Work out the finished part from the listing and answer in its coordinate system (mm). Face numbers are marked on the shaded views. A direction names the side the tool comes from. Coordinates: 2 decimals unless noted, no trailing zeros. Use a Markdown table: item, result.
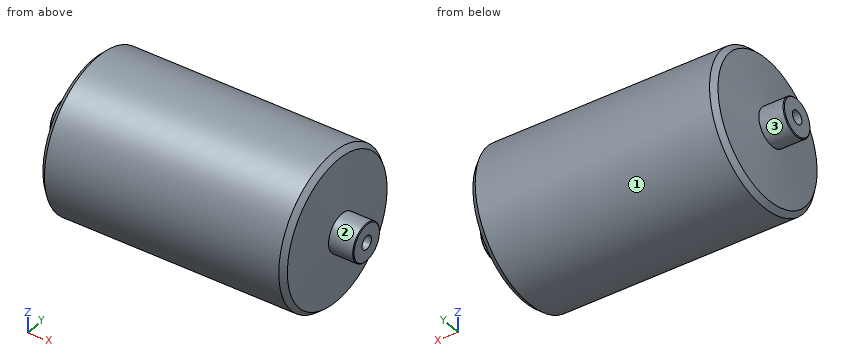
from build123d import *
from OCP.BRepFilletAPI import BRepFilletAPI_MakeChamfer

# Parameters (mm, degrees)
SKETCH_1_W       = 16.4
SKETCH_1_H       = 12.5
SKETCH_1_W_2     = 16.5
CHAMFER_1_SIZE   = 0.5
CHAMFER_2_SIZE   = 3
CHAMFER_2_SIZE2  = 3.300188603
M10X1_25_1_D     = 8.8
M10X1_25_1_DEPTH = 59
M10X1_25_1_TIP   = 2.643786724
M10X1_25_2_D     = 8.8
M10X1_25_2_DEPTH = 59
M10X1_25_2_TIP   = 2.643786724


with BuildPart() as part:
    # 草圖1 → 旋轉1 (revolve)
    with BuildSketch(Plane.XY, mode=Mode.PRIVATE) as revolve_1_sk:
        Polygon((16.5, 12.5), (16.5, 0), (183.6, 0), (183.6, 12.5), (183.6, 50), (16.5, 50), align=None)
        with Locations((191.8, 6.25)):
            Rectangle(SKETCH_1_W, SKETCH_1_H)
        with Locations((8.25, 6.25)):
            Rectangle(SKETCH_1_W_2, SKETCH_1_H)
    revolve(revolve_1_sk.sketch.rotate(Axis((16.5, 0, 0), (1, 0, 0)), 90), axis=Axis((16.5, 0, 0), (1, 0, 0)))

    # 草圖2 → 除料-旋轉1 (revolve, cut)
    with BuildSketch(Plane.XY, mode=Mode.PRIVATE) as cut_revolve_1_sk:
        Polygon((186.873055919, 74.843370729), (1.025224849, 63.173855755), (0, 12.5), (16.5, 12.5), (20.558049953, 58.883723216), (178.981866404, 65.285508546), (183.6, 12.5), (200, 12.5), align=None)
    revolve(cut_revolve_1_sk.sketch.rotate(Axis((0, 0, 0), (-1, 0, 0)), 270), axis=Axis((0, 0, 0), (-1, 0, 0)), mode=Mode.SUBTRACT)

    # 導角1
    chamfer_1_edges = [part.edges().sort_by_distance(p)[0] for p in [
        (200, 0, -12.5),
        (0, 0, -12.5),
    ]]
    chamfer(chamfer_1_edges, length=CHAMFER_1_SIZE)

    # 導角2: one chamfer whose edges measure the first distance from different faces: ONE call of the kernel's chamfer builder (chamfer() names one face for all edges)
    chamfer_2_edges_1 = [part.edges().sort_by_distance(p)[0] for p in [
        (19.780824882, 0, -50),
    ]]
    chamfer_2_side_1 = [part.faces().sort_by_distance(p)[0] for p in [
        (100.05, 0, -50),
    ]]
    chamfer_2_edges_2 = [part.edges().sort_by_distance(p)[0] for p in [
        (180.319175118, 0, -50),
    ]]
    chamfer_2_side_2 = [part.faces().sort_by_distance(p)[0] for p in [
        (181.959587559, 0, -31.25),
    ]]
    chamfer_2 = BRepFilletAPI_MakeChamfer(part.part.solid().wrapped)
    for e in chamfer_2_edges_1:
        chamfer_2.Add(CHAMFER_2_SIZE, CHAMFER_2_SIZE2, e.wrapped, chamfer_2_side_1[0].wrapped)  # the first distance lies on this face
    for e in chamfer_2_edges_2:
        chamfer_2.Add(CHAMFER_2_SIZE, CHAMFER_2_SIZE2, e.wrapped, chamfer_2_side_2[0].wrapped)  # the first distance lies on this face
    add(Compound.cast(chamfer_2.Shape()), mode=Mode.REPLACE)

    # M10x1.25 螺紋孔1
    with Locations(Plane(origin=(200, 0, 0), x_dir=(0, 0, 1), z_dir=(1, 0, 0))):
        with Locations((0, 0)):
            Hole(M10X1_25_1_D / 2, depth=M10X1_25_1_DEPTH)
            with Locations((0, 0, -(M10X1_25_1_DEPTH + M10X1_25_1_TIP / 2))):  # 118° drill point
                Cone(0, M10X1_25_1_D / 2, M10X1_25_1_TIP, mode=Mode.SUBTRACT)

    # M10x1.25 螺紋孔2
    with Locations(Plane.ZY):
        with Locations((0, 0)):
            Hole(M10X1_25_2_D / 2, depth=M10X1_25_2_DEPTH)
            with Locations((0, 0, -(M10X1_25_2_DEPTH + M10X1_25_2_TIP / 2))):  # 118° drill point
                Cone(0, M10X1_25_2_D / 2, M10X1_25_2_TIP, mode=Mode.SUBTRACT)


solid = part.part
Q1. Consider line 1 (Y direction, x = 163, z = 0); line 2 (Y direction, x = 101, z = -1); line 3 (Z direction, x = 160, y = 3). Determine where each line is inside the solid, lowest interval first. Write a range as [from, to].
Solved:
| item | result |
|---|---|
| line 1 | [-50, -4.4], [4.4, 50] |
| line 2 | [-49.99, 49.99] |
| line 3 | [-49.91, -3.22], [3.22, 49.91] |
Q2. Given pin 1 Ø2 at (x, z) = (118.5, -9) entering from +Y; pin 2 Ø10 at (x, z) = (146.5, 10) entering from +Y; pin 3 Ø3 at (x, y) = (178.5, 27) entering from -Z, each flat-ended and moving along its own axis, determine where each tip first touches the part or whether it passes through.
Solved:
| item | result |
|---|---|
| pin 1 | y = 49.36 |
| pin 2 | y = 49.75 |
| pin 3 | z = -42.38 |
Q3. For the marked faces 1, 2 and 3, determine the directions among +Z, -Z, +X, -X, +Y, -Y from which every point of the face is accessible in a straight line to the end or side of a thin tool.
Solved:
| item | result |
|---|---|
| face 1 | +X, -X |
| face 2 | +X |
| face 3 | -X |
